```python
from build123d import *
from build123d.topology import SkipClean

# Parameters (mm, degrees)
BOSS_EXTRUDE1_DEPTH = 4
SKETCH2_R           = 256
CUT_EXTRUDE1_DEPTH  = 4
SKETCH3_R           = 258
SKETCH3_R_2         = 256
EXTRUDE_THIN1_DEPTH = 10
SKETCH5_R           = 4
BOSS_EXTRUDE2_DEPTH = 30
CIRPATTERN1_COUNT   = 12


with BuildPart() as part:
    # Sketch1 → Boss-Extrude1 (new body)
    with BuildSketch(Plane.XY):
        with BuildLine():
            Line((865.269127642, 521.057153497), (865.269127642, 757.057153497))
            ThreePointArc((865.269127642, 757.057153497), (782.812941082, 1010.7278743), (545.269127642, 1132.057153497))
            ThreePointArc((545.269127642, 1132.057153497), (233.519744905, 1040.749713195), (75.269127642, 757.057153497))
            ThreePointArc((75.269127642, 757.057153497), (198.687627947, 391.283260157), (545.269127642, 221.271697797))
            ThreePointArc((545.269127642, 221.271697797), (725.219790584, 211.189307063), (905.269127642, 203.057153497))
            Line((905.269127642, 203.057153497), (905.269127642, 521.057153497))
            Line((905.269127642, 521.057153497), (865.269127642, 521.057153497))
        make_face()
    extrude(amount=BOSS_EXTRUDE1_DEPTH)

    # Sketch2 → Cut-Extrude1 (cut)
    with BuildSketch(Plane.XY.offset(4)):
        with Locations((545.269127642, 758.057153497)):
            Circle(SKETCH2_R)
    extrude(amount=-CUT_EXTRUDE1_DEPTH, mode=Mode.SUBTRACT)

    # Sketch3 → Extrude-Thin1 (add)
    with SkipClean():  # the faces are left unmerged after this step: merging them gives an invalid solid
        with BuildSketch(Plane(origin=(0, 0, 0), x_dir=(-1, 0, 0), z_dir=(0, 0, -1))):
            with Locations((-545.269127642, 758.057153497)):
                Circle(SKETCH3_R)
            with Locations((-545.269127642, 758.057153497)):
                Circle(SKETCH3_R_2, mode=Mode.SUBTRACT)
        extrude(amount=EXTRUDE_THIN1_DEPTH)
    add(part.part.scale(1), mode=Mode.REPLACE)  # the faces are merged on a copy

    # Sketch5 → Boss-Extrude2 (add)
    with BuildSketch(Plane.XY.offset(4)):
        with Locations(Location((545.269127642, 1033.057153497, 0), (0, 0, 180))):
            Circle(SKETCH5_R)
    boss_extrude2 = extrude(amount=BOSS_EXTRUDE2_DEPTH)

    # CirPattern1: Boss-Extrude2 ×12 about axis
    cirpattern1_axis = Axis((545.269127642, 758.057153497, 0), (0, 0, 1))
    for i in range(1, CIRPATTERN1_COUNT):
        add(boss_extrude2.rotate(cirpattern1_axis, i * 360 / CIRPATTERN1_COUNT))


solid = part.part
```
Geometry: final body of the model. Coordinates: model frame, mm. Give positions to 0.01 mm unless a question says otherwise; leave off trailing zeros. Order: outer loops, then holes, each group sorted by start corner. A loop starts at its lowest first (then second) coordinate and runs counter-clockwise, first axis right, second up. Notation, with made-up numbers: (21.5, -23.75) -> (49.5, -23.75) arc R25 ccw to (49.5, -8.75) -> close; hole circle Ø8 at (51.25, -17.5). An arc over 180 degrees is marked (long way). Write each question's results on one line, items separated by ' | '. Start each with the question number.
1) Line query: line 1 (Z direction, x = 748.5, y = 361); line 2 (Y direction, x = 631, z = -4.5); line 3 (X direction, y = 908.5, z = 1). Output: solid intervals per line, ascending. Write a range as from..to.
2) Section B-B (z = 22.5). Count the separate pieces of the cut face and the enclosed holes in it, then the cut area to 3 significant figures.
3) Section D-D (y = 262). Return loops of the section in (x, z), then the cut area to 3 significant figures.
4) Section C-C (y = 551.5). Return loops of the section in (x, z), then the cut area to 3 significant figures.
5) Section A-A (x = 427). Return loops of the section in (y, z), then the cut area to 3 significant figures.
6) First-contact query: pin 1 (6 mm diameter, centred on x = 754, z = -3.5, fed in from -Y); pin 2 (5 mm diameter, centred on y = 920.5, z = 3.5, fed in from +X); pin 3 (1.5 mm diameter, centred on y = 814, z = -4.5, fed in from +X). Flat tips, straight axial feed; report the tip coordinate or a pass-through.
Calculated:
1) line 1: 0..4 | line 2: 514.72..516.84, 999.28..1001.4 | line 3: 123.22..338.14, 752.4..843.44
2) separate pieces: 12 | enclosed holes: 0 | area: 603 mm2
3) outline: (375.81, 0) -> (905.27, 0) -> (905.27, 4) -> (375.81, 4) -> close | area: 2,120 mm2
4) outline: (104.03, 0) -> (390.68, 0) -> (390.68, -10) -> (394.04, -10) -> (394.04, 4) -> (104.03, 4) -> close; (696.5, -10) -> (699.86, -10) -> (699.86, 0) -> (865.27, 0) -> (865.27, 4) -> (696.5, 4) -> close | area: 1,900 mm2
5) outline: (242.97, 0) -> (528.76, 0) -> (528.76, -10) -> (531.01, -10) -> (531.01, 4) -> (242.97, 4) -> close; (985.1, -10) -> (987.35, -10) -> (987.35, 0) -> (1127.93, 0) -> (1127.93, 4) -> (985.1, 4) -> close | area: 1,770 mm2
6) pin 1: y = 602.37 | pin 2: x = 839.66 | pin 3: x = 797.3
